Input: part model. Units: mm. Frame: model coordinates. A direction names the side the tool comes from. Round coordinates to 2 decimals unless told otherwise and drop trailing zeros. Order: outer loops, then holes, each group sorted by start corner. A loop starts at its lowest first (then second) coordinate and runs counter-clockwise, first axis right, second up. Notation, with made-up numbers: (35.5, 10) - (70.5, 10) arc R13 ccw to (70.5, 22) - close; hole circle Ø2 at (-11, 71.5). An arc over 180 degrees is marked (long way). One line per item, written item: value. Start each with the question number.
from build123d import *

# Parameters (mm, degrees)
SKETCH1_R          = 15
SKETCH1_R_2        = 1.1
BASE_FLANGE1_DEPTH = 1


# Sheet-metal steps are written as plain solids
with BuildPart() as part:
    # Sketch1 → Base-Flange1 (new body)
    with BuildSketch(Plane.XY):
        Circle(SKETCH1_R)
        with Locations((0, 9.5)):
            Circle(SKETCH1_R_2, mode=Mode.SUBTRACT)
        with Locations((0, -9.5)):
            Circle(SKETCH1_R_2, mode=Mode.SUBTRACT)
        Polygon((1.59, 0), (1.59, 1.59), (-1.59, 1.59), (-1.59, -1.59), (1.59, -1.59), align=None, mode=Mode.SUBTRACT)
    extrude(amount=-BASE_FLANGE1_DEPTH)


solid = part.part
1. Section A-A (z = -0.4). Return the cut outline in (x, y), then the cut area to 3 significant figures.
2. Set-up query: faces 4 (the face through (3, 0, -1)), 5 (the face through (0, -1.59, -0.5)). Return all of +Z, -Z, +X, -X, +Y, -Y with unobstructed straight access to the full face (end or side cutting, diameter ignored); none if empty.
3. Line query: line 1 (Y direction, x = 0, z = -0.25); line 2 (X direction, y = -0.5, z = -0.9); line 3 (Y direction, x = -1.5, z = -0.85). Output: solid intervals per line, ascending. Write a range as from..to.
4. Section D-D (x = -11). Return the cut outline in (y, z).
5. Section C-C (y = 0). Return the cut outline in (x, z), then the cut area to 3 significant figures.
6. Section B-B (x = 0). Return the cut outline in (y, z), then the cut area to 3 significant figures.
7. Pull-direction query (X, two-part tool) for faces 1 (the face through (3, 0, 0)), 2 (the face through (-14.985, 0.66, -0.493)), 3 (the face through (-0.238, -10.574, -0.493)); classes: released by +X, released by -X, zero draft, split by the parting line, or undercut.
Solved:
1. outline: circle Ø30 at (0, 0); hole (-1.59, -1.59) - (1.59, -1.59) - (1.59, 1.59) - (-1.59, 1.59) - close; hole circle Ø2.2 at (0, -9.5); hole circle Ø2.2 at (0, 9.5)
1. area: 689 mm²
2. face 4: -Z, +X, -X, +Y, -Y
2. face 5: +Z, -Z
3. line 1: y = -15..-10.6, -8.4..-1.59, 1.59..8.4, 10.6..15
3. line 2: x = -14.99..-1.59, 1.59..14.99
3. line 3: y = -14.92..-1.59, 1.59..14.92
4. outline: (-10.2, -1) - (10.2, -1) - (10.2, 0) - (-10.2, 0) - close
5. outline: (-15, -1) - (-1.59, -1) - (-1.59, 0) - (-15, 0) - close; (1.59, -1) - (15, -1) - (15, 0) - (1.59, 0) - close
5. area: 26.8 mm²
6. outline: (-15, -1) - (-10.6, -1) - (-10.6, 0) - (-15, 0) - close; (-8.4, -1) - (-1.59, -1) - (-1.59, 0) - (-8.4, 0) - close; (1.59, -1) - (8.4, -1) - (8.4, 0) - (1.59, 0) - close; (10.6, -1) - (15, -1) - (15, 0) - (10.6, 0) - close
6. area: 22.4 mm²
7. face 1: zero draft
7. face 2: split by the parting line
7. face 3: undercut
